The model under review builds one solid part; all positions refer to its coordinate system, in mm. Face numbers are marked on the shaded views. A direction names the side the tool comes from. Coordinates: 2 decimals unless noted, no trailing zeros. Loops run counter-clockwise (first coordinate to the right, second up) from the corner with the lowest first, then second, coordinate; pieces in that order, holes last. Notation, with made-up numbers: M 18.5,15 L 77.5,15 A26 ccw 77.5,30 Z; hole C 54,-21.75 d5. An arc over 180 degrees is marked long. Write item = value, one per line. Start each with the question number.
Q1. We need section B-B on x = -1. Give the boundary of the cut face in (y, z).
Q2. We need section C-C on y = -24.5. Give the boundary of the cut face in (x, z).
Q3. Clearance check with flat-ended pins moving along their axes: pin 1 Ø12 at (y, z) = (-10.5, 9) entering from -X; pin 2 Ø11.5 at (y, z) = (-26, 30) entering from -X; pin 3 Ø10 at (y, z) = (-31.5, -29.5) entering from +X; pin 4 Ø20.5 at (x, y) = (6.5, -32.5) entering from +Z. State where each tip first meets the part, or that it passes through.
Q4. We need section A-A on y = -19. Give the boundary of the cut face in (x, z).
Q5. We need section D-D on z = -27.5. Give the boundary of the cut face in (x, y), and give its area (3 significant figures).
Q6. Mouldability with a two-part tool opening along X and no side actions: class the marked faces 6, 7 and 8 as released by +X, released by -X, zero draft, split by the parting line, or undercut.
Q7. Wall thickness on probe 1 along Z at (x, y) = (3, -37); probe 2 along Z at (x, y) = (-0.5, -30); probe 3 along Y at (x, z) = (47.5, -20): over which ranges is each line inside the solid? List them lowest first.
Q8. For the marked faces 1, 2, 3, 4 and 5, list the 3-axis set-ups (+Z, -Z, +X, -X, +Y, -Y) from which the entire face can be reached by the end or side of a thin tool; tool diameter is ignored.
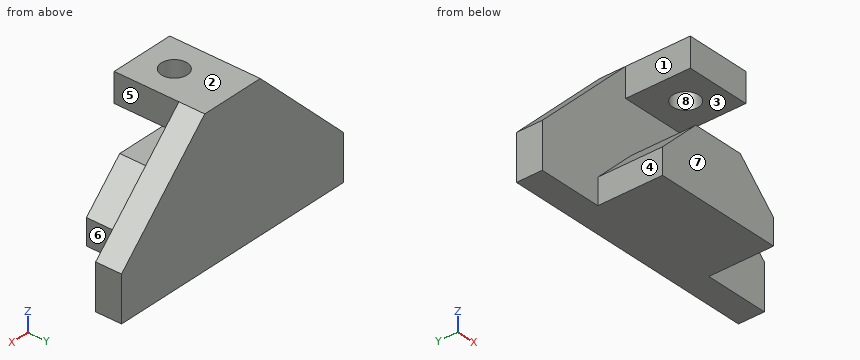
from build123d import *

# Parameters (mm, degrees)
F1_DEPTH = 12.7
F0_W     = 31.75
F0_H     = 14.2875
F2_DEPTH = 44.45
F3_R     = 6.35
F4_DEPTH = 25.4


with BuildPart() as f1:
    # F0 (on Front) → F1 (new body)
    with BuildSketch(Plane.XZ):
        Polygon((-60.109556, -13.391696), (-60.109556, -35.616696), (-28.359556, -35.616696), (-28.359556, -22.916696), (-9.309556, -3.866696), (16.090444, -3.866696), (35.140444, -22.916696), (35.140444, -35.616696), (66.890444, -35.616696), (66.890444, -13.391696), (19.265444, 34.233304), (19.265444, 19.945804), (-12.484556, 19.945804), (-12.484556, 34.233304), align=None)
    extrude(amount=F1_DEPTH)

    # F0 (on Front) → F2 (join)
    with BuildSketch(Plane.XZ):
        Polygon((-28.359556, -22.916696), (-28.359556, -35.616696), (-12.484556, -35.616696), (19.265444, -35.616696), (35.140444, -35.616696), (35.140444, -22.916696), (16.090444, -3.866696), (-9.309556, -3.866696), align=None)
        with Locations((3.390444, 27.089554)):
            Rectangle(F0_W, F0_H)
    extrude(amount=F2_DEPTH)

    # F3 (on face) → F4 (cut)
    with BuildSketch(Plane.XY.offset(34.233304)):
        with Locations((3.390444, -28.575)):
            Circle(F3_R)
    extrude(amount=-F4_DEPTH, mode=Mode.SUBTRACT)


solid = f1.part
Returned:
q1.outline = M -44.45,-35.62 L 0,-35.62 L 0,34.23 L -23.99,34.23 L -23.99,19.95 L -12.7,19.95 L -12.7,-3.87 L -44.45,-3.87 Z; M -44.45,19.95 L -33.16,19.95 L -33.16,34.23 L -44.45,34.23 Z
q2.outline = M -28.36,-35.62 L 35.14,-35.62 L 35.14,-22.92 L 16.09,-3.87 L -9.31,-3.87 L -28.36,-22.92 Z; M -12.48,19.95 L -1.48,19.95 L -1.48,34.23 L -12.48,34.23 Z; M 8.26,19.95 L 19.27,19.95 L 19.27,34.23 L 8.26,34.23 Z
q3.pin_1 = -43.72
q3.pin_2 = -12.48
q3.pin_3 = 35.14
q3.pin_4 = 34.23
q4.outline = M -28.36,-35.62 L 35.14,-35.62 L 35.14,-22.92 L 16.09,-3.87 L -9.31,-3.87 L -28.36,-22.92 Z; M -12.48,19.95 L 19.27,19.95 L 19.27,34.23 L -12.48,34.23 Z
q5.outline = M -60.11,-12.7 L -28.36,-12.7 L -28.36,-44.45 L 35.14,-44.45 L 35.14,-12.7 L 66.89,-12.7 L 66.89,0 L -60.11,0 Z
q5.area = 3,630 mm^2
q6.face_6 = released by +X
q6.face_7 = zero draft
q6.face_8 = undercut
q7.probe_1 = -35.62 to -3.87, 19.95 to 34.23
q7.probe_2 = -35.62 to -3.87
q7.probe_3 = -12.7 to 0
q8.face_1 = +Z, -X, -Y
q8.face_2 = +Z, +X, -X, +Y, -Y
q8.face_3 = +X, -X, -Y
q8.face_4 = +Z, -Z, -X, -Y
q8.face_5 = +Z, +X, -Y
